```python
from build123d import *

# Parameters (mm, degrees)
F0_R     = 20
F1_DEPTH = 60
F0_R_2   = 30
F2_DEPTH = 40
F3_R     = 5
F4_R     = 5
F5_R     = 4.99999


# Not quite as in the source:
# - a fillet or chamfer is up to 0.001 mm smaller than in the source, because OpenCascade refuses the exact size


with BuildPart() as f1:
    # F0 (on Top) → F1 (new body)
    with BuildSketch(Plane.XY):
        Circle(F0_R)
    extrude(amount=F1_DEPTH)

    # F0 (on Top) → F2 (join)
    with BuildSketch(Plane.XY):
        Circle(F0_R_2)
        Circle(F0_R, mode=Mode.SUBTRACT)
        Circle(F0_R)
    extrude(amount=-F2_DEPTH)

    # F3
    f3_edges = [f1.edges().sort_by_distance(p)[0] for p in [
        (-20, 0, 60),
    ]]
    fillet(f3_edges, radius=F3_R)

    # F4
    f4_edges = [f1.edges().sort_by_distance(p)[0] for p in [
        (-30, 0, 0),
    ]]
    fillet(f4_edges, radius=F4_R)

    # F5 (radius 5 in the source; OpenCascade refuses exactly that, so slightly less here)
    f5_edges = [f1.edges().sort_by_distance(p)[0] for p in [
        (-20, 0, 0),
    ]]
    fillet(f5_edges, radius=F5_R)


solid = f1.part
```
CAD build for the part. Positions are in the model's coordinates, mm. A direction names the side the tool comes from. Coordinates: 2 decimals unless noted, no trailing zeros. Loops run counter-clockwise (first coordinate to the right, second up) from the corner with the lowest first, then second, coordinate; pieces in that order, holes last. Notation, with made-up numbers: (-39.75, 88) - (14.25, 88) arc R7 cw to (14.25, 101) - close; hole circle Ø10 at (6, -9). An arc over 180 degrees is marked (long way). Return JSON: item names as keys, results as strings.
1. Band-saw the part on C-C (z = -13). Give the cut face in (x, y), and give its area (3 significant figures).
Result:
{"outline": "circle Ø60 at (0, 0)", "area": "2,830 mm2"}
2. 3-axis set-ups, long thin cutter, end or side, ignore diameter. For faces 1 (the flat face through (0, 0, -40)), 2 (the cylindrical face through (-4.336, -19.524, 29.65)): which of +Z, -Z, +X, -X, +Y, -Y reach the whole face in a straight line?
Result:
{"face 1": "-Z, +X, -X, +Y, -Y", "face 2": "+Z"}
3. Drop flat-ended pins along their axis: pin 1 (1 mm diameter, centred on x = -6, z = 47, fed in from -Y); pin 2 (2 mm diameter, centred on y = -20, z = -8, fed in from +X); pin 3 (1 mm diameter, centred on y = -12, z = -28, fed in from +X); pin 4 (12 mm diameter, centred on y = -1, z = -1.5, fed in from -X). Give the stop position or say it passes through.
Result:
{"pin 1": "stops at y = -19.23", "pin 2": "stops at x = 23.22", "pin 3": "stops at x = 27.71", "pin 4": "stops at x = -30"}
4. Probe L1, parallel to Z at x = 8.5, y = 12.5; L2, parallel to Z at x = -21, y = -14; L3, parallel to X at y = -25.5, z = -7. List the from-to ranges inside material, lowest first. Write a range as from..to.
Result:
{"L1": "z = -40..60", "L2": "z = -40..-0.01", "L3": "x = -15.8..15.8"}
